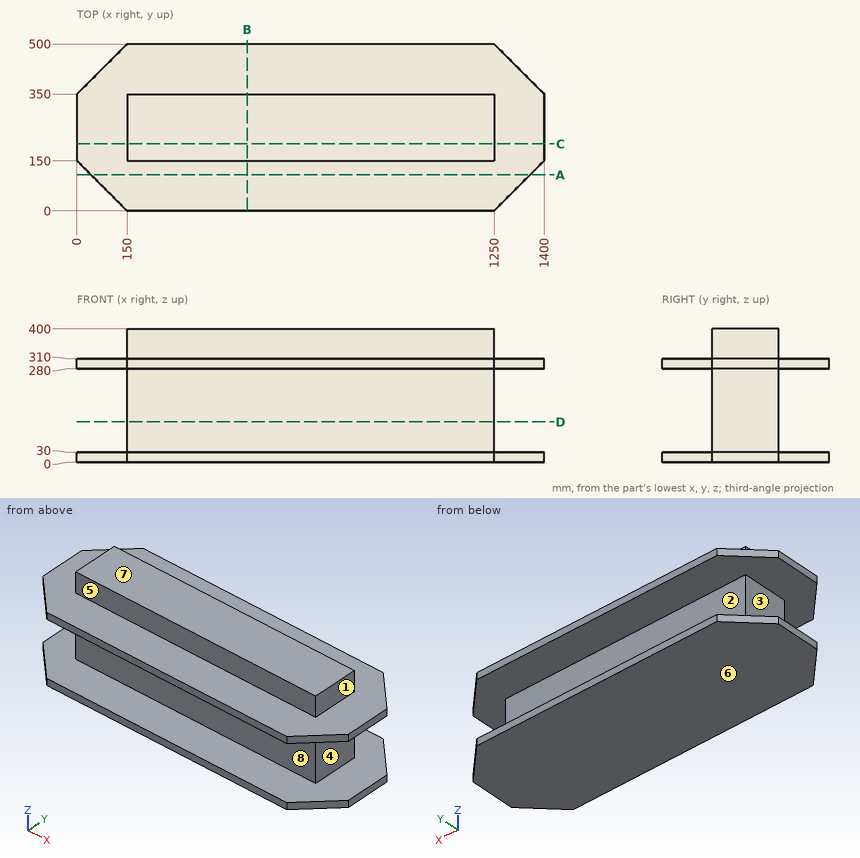
Print and shaded views of the part. All mm, measured from the part's lowest x, y and z. A direction names the side the tool comes from. Coordinates: 2 decimals unless noted, no trailing zeros. Write each loop counter-clockwise with the first axis right and the second up, starting at its lowest first coordinate (ties: lowest second). Pieces come first, ordered by that corner, then holes.
(1) Flat gauge pins, fed straight in: pin 1 (1.5 mm diameter, centred on x = 161, y = 69, fed in from +Z); pin 2 (10 mm diameter, centred on x = 1053, z = 208, fed in from +Y). Where does each tip first touch, or does it go through?
(2) Cut at B-B, the plane x = 509.5. List the corners of the cut face in (y, z).
(3) 3-axis set-ups, long thin cutter, end or side, ignore diameter. For the marked faces 1, 2, 3 and 4: which of +Z, -Z, +X, -X, +Y, -Y reach the whole face in a straight line?
(4) Cut at A-A, the plane y = 108. List the corners of the cut face in (x, z).
(5) Two-plate mould, pull along Z, no slides. Class the marked faces 5, 6, 7 and 8: +Z half, -Z half, draft (parallel to the pull), parting line (faces both ways), or undercut.
(6) Cut at C-C, the plane y = 200.5. List the corners of the cut face in (x, z), and give its area (3 significant figures).
(7) Cut at D-D, the plane z = 121. List the corners of the cut face in (x, y).
(8) Drill centre lines: probe 1 along Z at (x, y) = (108.5, 408); probe 2 along Y at (x, z) = (973.5, 41); probe 3 along Y at (x, z) = (123, 306). Where is each one in solid material? Low to high.
Geometry says:
1. pin 1: stops at z = 310
1. pin 2: stops at y = 350
2. outline: (0, 0) - (500, 0) - (500, 30) - (350, 30) - (350, 280) - (500, 280) - (500, 310) - (350, 310) - (350, 400) - (150, 400) - (150, 310) - (0, 310) - (0, 280) - (150, 280) - (150, 30) - (0, 30) - close
3. face 1: +Z, +X, +Y, -Y
3. face 2: +X, -X, +Y
3. face 3: -X, +Y, -Y
3. face 4: +X, +Y, -Y
4. outline: (42, 0) - (1358, 0) - (1358, 30) - (42, 30) - close; (42, 280) - (1358, 280) - (1358, 310) - (42, 310) - close
5. face 5: draft
5. face 6: -Z half
5. face 7: +Z half
5. face 8: undercut
6. outline: (0, 0) - (1400, 0) - (1400, 30) - (1250, 30) - (1250, 280) - (1400, 280) - (1400, 310) - (1250, 310) - (1250, 400) - (150, 400) - (150, 310) - (0, 310) - (0, 280) - (150, 280) - (150, 30) - (0, 30) - close
6. area: 458,000 mm2
7. outline: (150, 150) - (1250, 150) - (1250, 350) - (150, 350) - close
8. probe 1: z = 0 to 30, 280 to 310
8. probe 2: y = 150 to 350
8. probe 3: y = 27 to 473
